Design review of the part built by this model. Coordinates are the model's own, in mm. A direction names the side the tool comes from. Coordinates: 2 decimals unless noted, no trailing zeros. Loops run counter-clockwise (first coordinate to the right, second up) from the corner with the lowest first, then second, coordinate; pieces in that order, holes last. Notation, with made-up numbers: M 47.25,40 L 105.25,40 A18 ccw 105.25,60 Z; hole C 19.5,3.5 d3. An arc over 180 degrees is marked long. Put each result on its own line as item: value. Start each with the question number.
(1) Clearance check with flat-ended pins moving along their axes: pin 1 (2 mm diameter, centred on y = -0.5, z = -8, fed in from -X); pin 2 (1 mm diameter, centred on x = 5.5, y = -0.5, fed in from +Z) (3 decimals). State where each tip first meets the part, or that it passes through.
(2) Take a section at C-C, the plane x = 6. Give the boundary of the cut face in (y, z) (3 decimals).
(3) The part is to be moulded in two halves that separate along Y. For faces 1 (the cylindrical face through (5.23, -10.88, -1.43)), 2 (the cylindrical face through (1.972, 3.484, 10.696)), 3 (the cylindrical face through (1.972, 10.442, 6.669)), 4 (the cylindrical face through (1.97, 9.57, -7.87)), say which applies: +Y half, -Y half, draft (parallel to the pull), parting line (faces both ways), or undercut.
(4) Take a section at B-B, the plane z = 0. Give the boundary of the cut face in (x, y) (3 decimals), then the cut area to 3 significant figures.
(5) For probe 1 along Z at (x, y) = (1.5, 9.75); probe 2 along Z at (x, y) = (1, -11.75); probe 3 along X at (y, z) = (9.5, 6), list the stretches that pass through material, from the lowest coordinate up. Write a range as [from, to].
(6) For faces 5 (the cylindrical face through (1.972, -3.116, 11.992)), 6 (the cylindrical face through (1.97, 10.46, -6.69)), 7 (the cylindrical face through (2, 8.2, -7.7)), list the 3-axis set-ups (+Z, -Z, +X, -X, +Y, -Y) from which the entire face can be reached by the end or side of a thin tool; tool diameter is ignored.
(7) Take a section at A-A, the plane x = 1.5. Count the separate pieces of the cut face and the enclosed holes in it, then the cut area to 3 significant figures.
```python
from build123d import *

# Parameters (mm, degrees)
BASPROSKE_W                  = 4
BASPROSKE_H                  = 13.5
TOOTHCUT_DEPTH               = 20.506409203
TEETHCUTS_COUNT              = 25
TEETHCUTS_ANGLE              = 345.6
BORSKE_R                     = 1.5
BORE_DEPTH                   = 50.0000508
ESQUISSE1_R                  = 4.015099064
BOSS_EXTRU_1_DEPTH           = 4
ESQUISSE3_R                  = 10.975
BOSS_EXTRU_2_DEPTH           = 2.5
ENL_V_MAT_EXTRU_1_DEPTH      = 20.500499542
ENL_V_MAT_EXTRU_1_DEPTH_BACK = 20.500499542
ESQUISSE2_R                  = 1
ESQUISSE4_R                  = 2
ENL_V_MAT_EXTRU_2_DEPTH      = 2.5


with BuildPart() as part:
    # BasProSke → Base-Revolve (revolve)
    with BuildSketch(Plane(origin=(0, 0, 0), x_dir=(1, 0, 0), z_dir=(0, 1, 0)), mode=Mode.PRIVATE) as base_revolve_sk:
        with Locations((2, 6.75)):
            Rectangle(BASPROSKE_W, BASPROSKE_H)
    revolve(base_revolve_sk.sketch.rotate(Axis((-10, 0, 0), (1, 0, 0)), 180), axis=Axis((-10, 0, 0), (1, 0, 0)))

    # TooCutSke → ToothCut (cut, through all)
    with BuildSketch(Plane(origin=(0, 0, 0), x_dir=(0, 0, -1), z_dir=(1, 0, 0))):
        with BuildLine():
            ThreePointArc((0.570809389, 11.23450834), (0, 11.249), (-0.570809389, 11.23450834))
            ThreePointArc((-0.570809389, 11.23450834), (-0.823468719, 12.39261054), (-1.341642157, 13.4586939))
            ThreePointArc((-1.341642157, 13.4586939), (0, 13.5254), (1.341642157, 13.4586939))
            ThreePointArc((1.341642157, 13.4586939), (0.823468719, 12.39261054), (0.570809389, 11.23450834))
        make_face()
    toothcut = extrude(amount=TOOTHCUT_DEPTH, mode=Mode.SUBTRACT)

    # TeethCuts: ToothCut ×25 about axis
    teethcuts_axis = Axis((-10, 0, 0), (1, 0, 0))
    for i in range(1, TEETHCUTS_COUNT):
        add(toothcut.rotate(teethcuts_axis, i * TEETHCUTS_ANGLE / (TEETHCUTS_COUNT - 1)), mode=Mode.SUBTRACT)

    # BorSke → Bore (cut, symmetric)
    with BuildSketch(Plane(origin=(0, 0, 0), x_dir=(0, 0, -1), z_dir=(1, 0, 0))):
        with Locations(Location((0, 0, 0), (0, 0, 180))):
            Circle(BORSKE_R)
    extrude(amount=BORE_DEPTH, both=True, mode=Mode.SUBTRACT)

    # Esquisse1 → Boss.-Extru.1 (add)
    with BuildSketch(Plane(origin=(4, 0, 0), x_dir=(0, 0, -1), z_dir=(1, 0, 0))):
        Circle(ESQUISSE1_R)
    extrude(amount=-BOSS_EXTRU_1_DEPTH)

    # Esquisse3 → Boss.-Extru.2 (add)
    with BuildSketch(Plane(origin=(4, 0, 0), x_dir=(0, 0, -1), z_dir=(1, 0, 0))):
        with Locations(Location((0, 0, 0), (0, 0, 180))):
            Circle(ESQUISSE3_R)
    extrude(amount=BOSS_EXTRU_2_DEPTH)

    # Esquisse2 → Enlèv. mat.-Extru.1 (cut, two sides: drawn at the far end of the back side and taken through both)
    with BuildSketch(Plane(origin=(4, 0, 0), x_dir=(0, 0, -1), z_dir=(1, 0, 0)).offset(-ENL_V_MAT_EXTRU_1_DEPTH_BACK)):
        with Locations((-7.775, 0)):
            Circle(ESQUISSE2_R)
        with Locations((7.775, 0)):
            Circle(ESQUISSE2_R)
    extrude(amount=ENL_V_MAT_EXTRU_1_DEPTH + ENL_V_MAT_EXTRU_1_DEPTH_BACK, mode=Mode.SUBTRACT)

    # Esquisse4 → Enlèv. mat.-Extru.2 (cut)
    with BuildSketch(Plane.ZY):
        with Locations((-7.775, 0)):
            Circle(ESQUISSE4_R)
        with Locations((7.775, 0)):
            Circle(ESQUISSE4_R)
    extrude(amount=-ENL_V_MAT_EXTRU_2_DEPTH, mode=Mode.SUBTRACT)


solid = part.part
```
Computed values:
1. pin 1: stops at x = 2.5
1. pin 2: stops at z = 10.975
2. outline: C 0,0 d21.95; hole C 0,-7.775 d2; hole C 0,7.775 d2
3. face 1: parting line
3. face 2: undercut
3. face 3: +Y half
3. face 4: undercut
4. outline: M 0,-13.5 L 4,-13.5 L 4,-10.975 L 6.5,-10.975 L 6.5,10.975 L 4,10.975 L 4,11.249 L 0,11.249 Z
4. area: 154 mm^2
5. probe 1: z = [-7.95, -6.04], [-5.61, 5.61], [6.04, 7.95]
5. probe 2: z = [-6.65, -5.86], [-3.79, -2.18], [-0.83, 0.83], [2.18, 3.79], [5.86, 6.65]
5. probe 3: x = [0, 4]
6. face 5: +Z, +X, -X
6. face 6: +X, -X, +Y
6. face 7: +X, -X
7. separate pieces: 1
7. enclosed holes: 2
7. area: 451 mm^2
